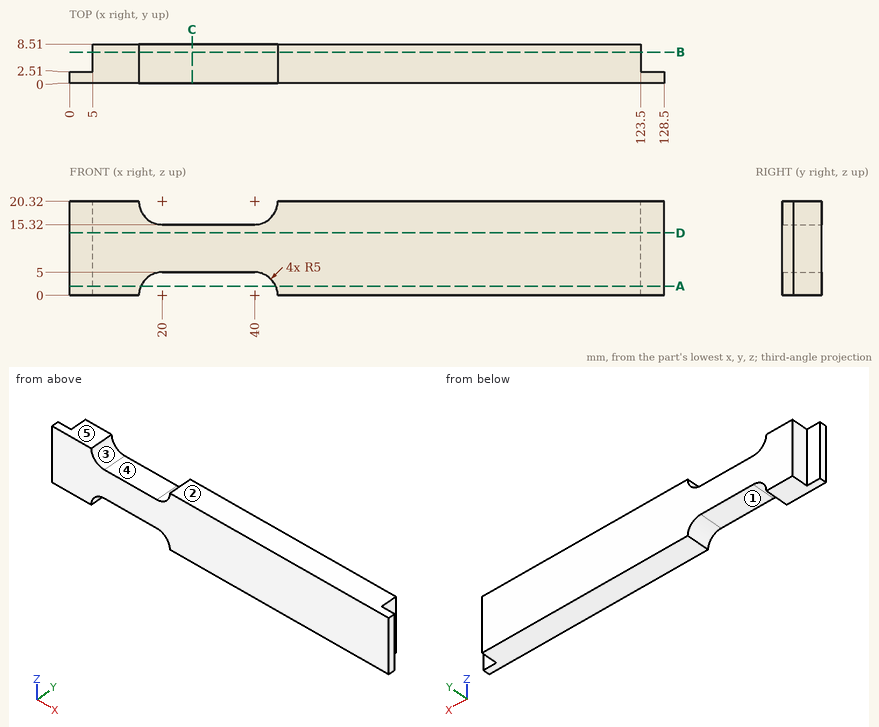
Geometry check sheet. Reference: drawing and pictorial views, mm from the part's lowest x, y, z. A direction names the side the tool comes from. Give positions to 0.01 mm unless a question says otherwise; leave off trailing zeros. Write each loop counter-clockwise with the first axis right and the second up, starting at its lowest first coordinate (ties: lowest second). Pieces come first, ordered by that corner, then holes.
Item 1: Cross-section at D-D (z = 13.5). Enter the section's corners in (x, y), and give its area (3 significant figures).
Item 2: Draft check along X on the marked faces 4 and 5. Enter one of: released by +X, released by -X, zero draft, split by the parting line, or undercut.
Item 3: Cross-section at C-C (x = 26.5). Enter the section's corners in (y, z), and give its area (3 significant figures).
Item 4: Scan lines: L1, parallel to X at y = 1, z = 16.5; L2, parallel to X at y = 6.5, z = 16.75; L3, parallel to X at y = 4.25, z = 6.25. Record each from-to range of solid material in increasing order.
Item 5: Cross-section at B-B (y = 6.75). Enter the section's corners in (x, z).
Item 6: Cross-section at A-A (z = 2). Enter the section's corners in (x, y).
Item 7: Gauge pin test, flat ends, axial feed: pin 1 (2.5 mm diameter, centred on x = 33, y = 2, fed in from +Z); pin 2 (5.5 mm diameter, centred on x = 126.5, z = 8.5, fed in from +Y); pin 3 (5 mm diameter, centred on y = 5.5, z = 10, fed in from -X). Record the tip position at first contact, or that the pin passes through.
Item 8: Access from +Z, -Z, +X, -X, +Y, -Y to the whole of each face (thin tool, end or side, straight path). Record for the marked faces 1, 2 and 3.
Report:
1. outline: (0, 0) - (128.5, 0) - (128.5, 2.51) - (123.5, 2.51) - (123.5, 8.51) - (5, 8.51) - (5, 2.51) - (0, 2.51) - close
1. area: 1,030 mm2
2. face 4: undercut
2. face 5: zero draft
3. outline: (0, 5) - (8.51, 5) - (8.51, 15.32) - (0, 15.32) - close
3. area: 87.8 mm2
4. L1: x = 0 to 16.77, 43.23 to 128.5
4. L2: x = 5 to 16.5, 43.5 to 123.5
4. L3: x = 5 to 123.5
5. outline: (5, 0) - (15, 0) arc R5 cw to (20, 5) - (40, 5) arc R5 cw to (45, 0) - (123.5, 0) - (123.5, 20.32) - (45, 20.32) arc R5 cw to (40, 15.32) - (20, 15.32) arc R5 cw to (15, 20.32) - (5, 20.32) - close
6. outline: (0, 0) - (15.42, 0) - (15.42, 8.51) - (5, 8.51) - (5, 2.51) - (0, 2.51) - close; (44.58, 0) - (128.5, 0) - (128.5, 2.51) - (123.5, 2.51) - (123.5, 8.51) - (44.58, 8.51) - close
7. pin 1: stops at z = 15.32
7. pin 2: stops at y = 2.51
7. pin 3: stops at x = 5
8. face 1: -Z, +Y, -Y
8. face 2: +Z, +X, -X, +Y, -Y
8. face 3: +Z, +Y, -Y
